Geometry check sheet. Reference: the model listing, model coordinates, mm. Face numbers are marked on the shaded views. A direction names the side the tool comes from. Round coordinates to 2 decimals unless told otherwise and drop trailing zeros. Order: outer loops, then holes, each group sorted by start corner. A loop starts at its lowest first (then second) coordinate and runs counter-clockwise, first axis right, second up. Notation, with made-up numbers: (35.25, 89) - (66.25, 89) arc R12 cw to (66.25, 103) - close; hole circle Ø7 at (51.25, -36.75). An arc over 180 degrees is marked (long way). Answer as CSV lines item,"result". Start each with the question number.
```python
from build123d import *

# Parameters (mm, degrees)
F0_W     = 65
F0_H     = 33
F0_W_2   = 54.1921891272
F0_H_2   = 23.9197313786
F1_DEPTH = 10
F2_T     = -1
F3_DEPTH = 73.8002602011


with BuildPart() as f1:
    # F0 (on Front) → F1 (new body)
    with BuildSketch(Plane.XZ):
        Rectangle(F0_W, F0_H)
        Rectangle(F0_W_2, F0_H_2, mode=Mode.SUBTRACT)
        Rectangle(F0_W_2, F0_H_2)
    extrude(amount=F1_DEPTH)

    # F2
    f2_openings = [f1.faces().sort_by_distance(p)[0] for p in [
        (0, -10, 0),
    ]]
    offset(amount=F2_T, openings=f2_openings)

    # F0 (on Front) → F3 (cut)
    with BuildSketch(Plane.XZ):
        Rectangle(F0_W_2, F0_H_2)
    extrude(amount=F3_DEPTH, mode=Mode.SUBTRACT)


solid = f1.part
```
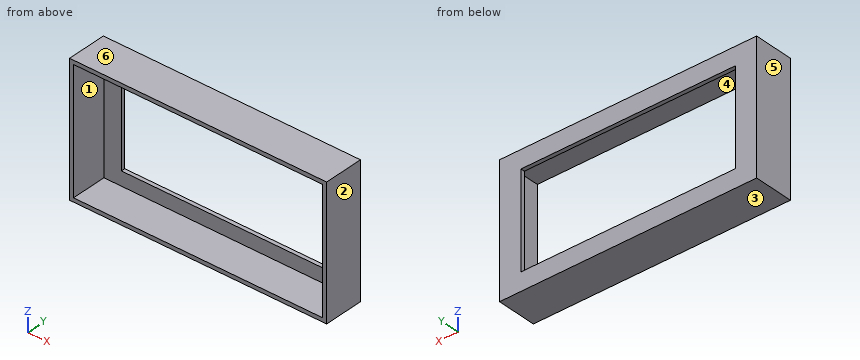
1. Access from +Z, -Z, +X, -X, +Y, -Y to the whole of each face (thin tool, end or side, straight path). Record for the marked faces 1 and 2.
2. Section check A-A on x = -2. Record the boundary of the cut face in (y, z).
3. Section check B-B on y = -2.75. Record the boundary of the cut face in (x, z), plus the area to 3 significant figures.
4. Thickness scan on probe 1 along Z at (x, y) = (-28.5, -9); probe 2 along X at (y, z) = (-8.25, -8); probe 3 along X at (y, z) = (-0.75, -10.5). Record the ranges inside material, lowest first.
5. Section check D-D on z = -13. Record the boundary of the cut face in (x, y), plus the area to 3 significant figures.
6. Draft check along Z on the marked faces 3, 4, 5 and 6. Enter one of: released by +Z, released by -Z, zero draft, split by the parting line, or undercut.
7. Section check C-C on z = -0.5. Record the boundary of the cut face in (x, y), plus the area to 3 significant figures.
Numbers:
1,face 1,"-Y"
1,face 2,"+Z, -Z, +X, +Y, -Y"
2,outline,"(-10, -16.5) - (0, -16.5) - (0, -11.96) - (-1, -11.96) - (-1, -15.5) - (-10, -15.5) - close; (-10, 15.5) - (-1, 15.5) - (-1, 11.96) - (0, 11.96) - (0, 16.5) - (-10, 16.5) - close"
3,outline,"(-32.5, -16.5) - (32.5, -16.5) - (32.5, 16.5) - (-32.5, 16.5) - close; hole (-31.5, -15.5) - (31.5, -15.5) - (31.5, 15.5) - (-31.5, 15.5) - close"
3,area,"192 mm2"
4,probe 1,"z = -16.5 to -15.5, 15.5 to 16.5"
4,probe 2,"x = -32.5 to -31.5, 31.5 to 32.5"
4,probe 3,"x = -32.5 to -27.1, 27.1 to 32.5"
5,outline,"(-32.5, -10) - (-31.5, -10) - (-31.5, -1) - (31.5, -1) - (31.5, -10) - (32.5, -10) - (32.5, 0) - (-32.5, 0) - close"
5,area,"83.0 mm2"
6,face 3,"released by -Z"
6,face 4,"undercut"
6,face 5,"zero draft"
6,face 6,"released by +Z"
7,outline,"(-32.5, -10) - (-31.5, -10) - (-31.5, -1) - (-27.1, -1) - (-27.1, 0) - (-32.5, 0) - close; (27.1, -1) - (31.5, -1) - (31.5, -10) - (32.5, -10) - (32.5, 0) - (27.1, 0) - close"
7,area,"28.8 mm2"
